Autodesk Inventor part; units mm, degrees
ref_plane "YZ Plane" through (0, 0, 0) normal (1, 0, 0) x (0, 1, 0)
ref_plane "XZ Plane" through (0, 0, 0) normal (0, 1, 0) x (-1, 0, 0)
ref_plane "XY Plane" through (0, 0, 0) normal (0, 0, 1) x (1, 0, 0)
sketch "Sketch1" plane through (0, 0, 0) normal (0, 1, 0) x (-1, 0, 0)
  circle A0 centre (0, 0) radius 1.65
  circle A1 centre (0, 0) radius 3
  circle A2 centre (5.12, 83.75) radius 1.65
  circle A3 centre (5.12, 83.75) radius 3
  circle A4 centre (93.53, 3.15) radius 1.65
  circle A5 centre (93.53, 3.15) radius 3
  line L0 (-6.58, 0) -> (-6.58, -6.22)
  line L1 (-6.58, -6.22) -> (-6.58, 91.53)
  line L2 (-6.58, 91.53) -> (103.15, 91.53)
  line L3 (103.15, 86.53) -> (103.15, -1.22)
  line L4 (103.15, -6.22) -> (-6.58, -6.22)
  line L5 (-6.58, 91.53) -> (-6.58, 88.53)
  line L6 (103.15, 91.53) -> (100.15, 91.53)
  line L7 (3, 0) -> (3, -3.22)
  line L8 (-3, 0) -> (-3, -3.22)
  line L9 (2.12, 83.75) -> (2.12, 88.53)
  line L10 (8.12, 83.75) -> (8.12, 88.53)
  line L11 (93.53, 6.15) -> (100.15, 6.15)
  line L12 (93.53, 0.15) -> (100.15, 0.15)
  line L13 (-3.58, 88.53) -> (-3.58, -3.22)
  line L14 (103.15, 91.53) -> (108.15, 91.53)
  line L15 (108.15, 91.53) -> (108.15, 86.53)
  line L16 (108.15, 86.53) -> (103.15, 86.53)
  line L17 (103.15, -6.22) -> (108.15, -6.22)
  line L18 (108.15, -6.22) -> (108.15, -1.22)
  line L19 (108.15, -1.22) -> (103.15, -1.22)
  line L20 (100.15, 88.53) -> (100.15, 6.15)
  line L21 (100.15, 0.15) -> (100.15, -3.22)
  line L22 (100.15, -3.22) -> (3, -3.22)
  line L23 (-3, -3.22) -> (-3.58, -3.22)
  line L24 (-3.58, 88.53) -> (2.12, 88.53)
  line L25 (8.12, 88.53) -> (100.15, 88.53)
  dimension "d0" = 3.3
  dimension "d1" = 6
  dimension "d4" = 3.3
  dimension "d5" = 6
  dimension "d8" = 3.3
  dimension "d9" = 6
extrude "Extrusion1" add sketch "Sketch1" against normal blind 3 contours A1 | A5 | A3 | L1 L2 L14 L15 L16 L3 L19 L18 L17 L4 L0
extrude "Extrusion2" add sketch "Sketch1" along normal blind 3 contours A1 | A5 | A3
sketch "Sketch2" plane through (0, 0, 0) normal (0, 1, 0) x (1, 0, 0)
  line L0 (-103.15, 1.22) -> (-108.15, 1.22)
  line L1 (-103.15, 1.22) -> (-103.15, 6.22)
  line L2 (-108.15, 6.22) -> (6.58, 6.22)
  line L3 (-103.15, 6.22) -> (-108.15, 6.22)
  line L4 (-108.15, 6.22) -> (-108.15, 1.22)
  line L5 (-103.15, 1.22) -> (-103.15, -86.53)
  line L6 (-108.15, 1.22) -> (-103.15, 1.22)
  line L7 (-108.15, -91.53) -> (-108.15, -86.53)
  line L8 (-108.15, -91.53) -> (-103.15, -91.53)
  line L9 (6.58, -91.53) -> (-108.15, -91.53)
  line L10 (-103.15, -86.53) -> (-103.15, -91.53)
  line L11 (-108.15, -86.53) -> (-103.15, -86.53)
  line L12 (-103.15, -86.53) -> (-108.15, -86.53)
  line L13 (-108.15, -86.53) -> (-108.15, -91.53)
  line L14 (-103.15, -91.53) -> (-104.15, -91.53)
  line L15 (-104.15, -91.53) -> (-104.15, -86.53)
  line L16 (-103.15, 1.22) -> (-104.15, 1.22)
  line L17 (-104.15, 1.22) -> (-104.15, 6.22)
  point P0 (0, 0)
  dimension "d26" = 1
  dimension "d27" = 1
extrude "Extrusion3" add sketch "Sketch2" along normal blind 41 contours L0 L4 L2 L17 | L15 L8 L7 L11
sketch "Sketch3" plane through (-104.15, 0, 91.53) normal (1, 0, 0) x (0, 0, -1)
  line L0 (0, 41) -> (5, 41)
  line L1 (0, 41) -> (0, 38)
  line L2 (0, -3) -> (0, 41)
  line L3 (0, 38) -> (5, 38)
  line L4 (5, -3) -> (5, 41)
  line L5 (5, 38) -> (5, 41)
  line L6 (5, 41) -> (0, 41)
  line L7 (92.75, 41) -> (97.75, 41)
  line L8 (92.75, 41) -> (92.75, 38)
  line L9 (92.75, -3) -> (92.75, 41)
  line L10 (92.75, 38) -> (97.75, 38)
  line L11 (97.75, -3) -> (97.75, 41)
  line L12 (97.75, 41) -> (92.75, 41)
  line L13 (97.75, 41) -> (97.75, 38)
  point P0 (91.53, 0)
  dimension "d30" = 3
  dimension "d31" = 3
extrude "Extrusion4" add sketch "Sketch3" along normal blind 35
sketch "Sketch4" plane through (0, 41, 0) normal (0, 1, 0) x (1, 0, 0)
  line L0 (-69.15, -91.53) -> (-69.15, -86.53)
  line L1 (-108.15, 1.22) -> (-69.15, 1.22)
  line L2 (-69.15, -86.53) -> (-69.15, -78.155)
  line L3 (-69.15, 1.22) -> (-69.15, -7.155)
  circle A0 centre (-74.23, -78.155) radius 1.65
  circle A1 centre (-74.23, -7.155) radius 1.65
  circle A2 centre (-92.01, -78.155) radius 1.65
  circle A3 centre (-92.01, -7.155) radius 1.65
  line L4 (-69.15, -78.155) -> (-69.15, -75.155)
  line L5 (-69.15, -75.155) -> (-69.15, -74.155)
  line L6 (-69.15, -74.155) -> (-97.09, -74.155)
  line L7 (-100.15, -88.53) -> (-100.15, -6.15)
  line L8 (-97.09, -74.155) -> (-97.09, -86.53)
  line L9 (-97.09, -86.53) -> (-69.15, -86.53)
  line L10 (-69.15, -7.155) -> (-69.15, -11.155)
  line L11 (-69.15, -11.155) -> (-97.09, -11.155)
  line L12 (-97.09, -11.155) -> (-97.09, 1.22)
  line L13 (-97.09, 1.22) -> (-69.15, 1.22)
  point P0 (0, 0)
  dimension "d46" = 3.3
  dimension "d47" = 3.3
  dimension "d50" = 3.3
  dimension "d51" = 3.3
  dimension "d53" = 1
extrude "Extrusion5" add sketch "Sketch4" against normal blind 3
sketch "Sketch5" plane through (-69.15, 0, 91.53) normal (1, 0, 0) x (0, 0, -1)
  line L0 (0, 41) -> (0, 38)
  line L1 (0, 41) -> (0, 38)
  line L2 (0, 41) -> (17.375, 41)
  line L3 (0, 41) -> (5, 41)
  line L4 (5, 41) -> (5, 38)
  line L5 (5, -3) -> (5, 41)
  line L6 (5, 38) -> (0, 38)
  line L7 (0, 38) -> (5, 38)
  line L8 (97.75, 38) -> (97.75, 41)
  line L9 (97.75, 41) -> (92.75, 41)
  line L10 (97.75, 41) -> (80.375, 41)
  line L11 (92.75, 38) -> (92.75, 41)
  line L12 (92.75, 41) -> (92.75, 38)
  line L13 (97.75, 38) -> (80.375, 38)
  line L14 (92.75, 38) -> (97.75, 38)
  line L15 (97.75, 38) -> (97.75, 41)
  point P0 (91.53, 0)
  dimension "d59" = 5
  dimension "d60" = 5
extrude "Extrusion6" add sketch "Sketch5" along normal blind 30
sketch "Sketch7" plane through (0, 41, 0) normal (0, 1, 0) x (1, 0, 0)
  line L0 (-69.15, 1.22) -> (-69.15, -11.155)
  line L1 (-69.15, 1.22) -> (-46.15, 1.22)
  line L2 (-3, 3.22) -> (-100.15, 3.22)
  line L3 (-69.15, 1.22) -> (-69.15, -11.155)
  line L4 (-69.15, -11.155) -> (-69.15, -25.405)
  line L5 (-69.15, -25.405) -> (-39.15, -25.405)
  line L6 (-39.15, 1.22) -> (-39.15, 6.22)
  line L7 (-39.15, -25.405) -> (-39.15, 1.22)
  line L8 (-39.15, 1.22) -> (-46.15, 1.22)
  circle A0 centre (-54.15, -17.905) radius 3.75
  point P0 (0, 0)
  dimension "d117" = 7.5
extrude "Extrusion8" add sketch "Sketch7" against normal blind 2
sketch "Sketch8" plane through (0, 41, 0) normal (0, 1, 0) x (1, 0, 0)
  circle A0 centre (-74.23, -78.155) radius 1.65
  circle A1 centre (-64.15, -68.155) radius 1
  circle A2 centre (-44.15, -68.155) radius 1
  circle A3 centre (-54.15, -38.155) radius 1
  line L0 (-39.15, -91.53) -> (-39.15, -86.53)
  line L1 (-39.15, -86.53) -> (-42.15, -86.53)
  line L2 (-42.15, -86.53) -> (-42.15, -39.155)
  line L3 (-42.15, -39.155) -> (-42.15, -36.155)
  line L4 (-66.15, -86.53) -> (-66.15, -36.155)
  line L5 (-66.15, -86.53) -> (-42.15, -86.53)
  line L6 (-66.15, -86.53) -> (-62.15, -86.53)
  line L7 (-69.15, -86.53) -> (-39.15, -86.53)
  line L8 (-42.15, -86.53) -> (-46.15, -86.53)
  line L9 (-62.15, -36.155) -> (-42.15, -36.155)
  line L10 (-62.15, -36.155) -> (-66.15, -36.155)
  line L11 (-46.15, -40.155) -> (-62.15, -40.155)
  line L12 (-62.15, -86.53) -> (-62.15, -40.155)
  line L13 (-46.15, -86.53) -> (-46.15, -40.155)
  point P0 (0, 0)
  dimension "d81" = 2
  dimension "d85" = 3
  dimension "d86" = 3
  dimension "d88" = 4
  dimension "d89" = 4
extrude "Extrusion9" add sketch "Sketch8" against normal blind 3 contours L5 L13 L11 L12 L4 L10 L9 L3 L2
sketch "Sketch9" plane through (0, 41, 0) normal (0, 1, 0) x (1, 0, 0)
  line L0 (-39.15, -91.53) -> (-36.15, -91.53)
  line L1 (-104.15, -91.53) -> (6.58, -91.53)
  line L2 (-36.15, -91.53) -> (-36.15, 6.22)
  line L3 (-108.15, 6.22) -> (6.58, 6.22)
  line L4 (-36.15, 6.22) -> (-39.15, 6.22)
  line L5 (-104.15, -91.53) -> (-39.15, -91.53)
  line L6 (-39.15, 6.22) -> (-39.15, -91.53)
  point P0 (0, 0)
  dimension "d94" = 3
extrude "Extrusion10" add sketch "Sketch9" against normal blind 3
sketch "Sketch10" plane through (0, 41, 0) normal (0, 1, 0) x (1, 0, 0)
  line L0 (-108.15, -86.53) -> (-103.15, -86.53)
  line L1 (-108.15, 6.22) -> (-108.15, 1.22)
  line L2 (-108.15, -86.53) -> (-108.15, 1.22)
  line L3 (-108.15, 1.22) -> (-105.15, 1.22)
  line L4 (-108.15, 1.22) -> (-97.09, 1.22)
  line L5 (-105.15, 1.22) -> (-105.15, -86.53)
  line L6 (-103.15, 1.22) -> (-103.15, -86.53)
  line L7 (-105.15, -86.53) -> (-108.15, -86.53)
  point P0 (0, 0)
  dimension "d97" = 3
extrude "Extrusion11" add sketch "Sketch10" against normal blind 3 contours L2 L3 L5 L0
sketch "Sketch11" plane through (0, 41, 0) normal (0, 1, 0) x (1, 0, 0)
  line L0 (-86.93, -78.155) -> (-86.93, -86.53)
  line L1 (-79.31, -78.155) -> (-79.31, -86.53)
  line L2 (-79.31, -86.53) -> (-86.93, -86.53)
  line L3 (-79.31, -78.155) -> (-79.31, -74.155)
  line L4 (-79.31, -74.155) -> (-86.93, -74.155)
  line L5 (-86.93, -78.155) -> (-86.93, -74.155)
  line L6 (-86.93, -7.155) -> (-86.93, 0)
  line L7 (-79.31, -7.155) -> (-79.31, 0)
  line L8 (-79.31, 0) -> (-86.93, 0)
  line L9 (-79.31, -7.155) -> (-79.31, -11.155)
  line L10 (-86.93, -7.155) -> (-86.93, -11.155)
  line L11 (-86.93, -11.155) -> (-79.31, -11.155)
  line L12 (-47.07, -17.905) -> (-47.07, 0)
  line L13 (-61.95, -17.905) -> (-61.95, 0)
  line L14 (-61.95, -17.905) -> (-61.95, -25.405)
  line L15 (-69.15, -25.405) -> (-39.15, -25.405)
  line L16 (-61.95, -25.405) -> (-47.07, -25.405)
  line L17 (-47.07, -25.405) -> (-47.07, -17.905)
  line L18 (-61.95, -25.405) -> (-69.15, -25.405)
  line L19 (-69.15, -25.405) -> (-69.15, 0)
  line L20 (-69.15, 1.22) -> (-69.15, -11.155)
  line L21 (-61.95, 0) -> (-69.15, 0)
  line L22 (-47.07, -25.405) -> (-39.15, -25.405)
  line L23 (-39.15, -25.405) -> (-39.15, 0)
  line L24 (-39.15, 0) -> (-47.07, 0)
  line L25 (-54.15, -17.905) -> (-54.15, -25.405)
  line L26 (-39.15, -25.405) -> (-69.15, -25.405)
  line L27 (-54.15, -25.405) -> (-54.15, -17.905)
  line L28 (-54.15, -17.905) -> (-54.15, -10.405)
  line L29 (-54.15, -10.405) -> (-58.15, -10.405)
  line L30 (-58.15, -10.405) -> (-58.15, 0)
  line L31 (-58.15, 0) -> (-50.15, 0)
  line L32 (-50.15, 0) -> (-50.15, -10.405)
  line L33 (-50.15, -10.405) -> (-54.15, -10.405)
  point P0 (0, 0)
  point P1 (-92.01, -78.155)
  point P2 (-74.23, -78.155)
  point P3 (-92.01, -7.155)
  dimension "d111" = 7.5
  dimension "d112" = 7.5
  dimension "d113" = 4
  dimension "d114" = 8
extrude "Extrusion12" cut sketch "Sketch11" against normal blind 10
properties part number "electronic_holder"
Can you work these out from the model? Positions are in its coordinate system, mm. A direction names the side the tool comes from. Give positions to 0.01 mm unless a question says otherwise; leave off trailing zeros. Order: outer loops, then holes, each group sorted by start corner. A loop starts at its lowest first (then second) coordinate and runs counter-clockwise, first axis right, second up. Notation, with made-up numbers: M 15,71 L 39,71 A25 cw 39,105 Z; hole C -14,-34 d5. An arc over 180 degrees is marked long. Use one line per item in the form item = value.
Item 1: If I drill on line 1 along Z through (x, y) = (-93.53, -0.4); line 2 along X through (y, z) = (39, 55.5); line 3 along Z through (x, y) = (-92, 39) (3 decimals), over which ranges is the centre line in solid material (lowest first)? Write a range as [from, to].
Values follow:
line_1 = [-6.22, -3.22], [0.15, 1.5], [4.8, 6.15], [88.53, 91.53]
line_2 = [-108.15, -105.15], [-66.15, -62.15], [-46.15, -42.15], [-39.15, -36.15]
line_3 = [-6.22, 5.505], [8.805, 11.155], [74.155, 76.505], [79.805, 91.53]
Item 2: If we section it at A-A, the plane y = 36.5: Write out the boundary of the cut face in (x, z).
Values follow:
outline = M -108.15,-6.22 L -104.15,-6.22 L -104.15,-1.22 L -108.15,-1.22 Z; M -108.15,86.53 L -104.15,86.53 L -104.15,91.53 L -108.15,91.53 Z
Item 3: Thinking about a two-plate mould opening in X: for faces 1 (the flat face through (-1.3, 3, -1.3)), 2 (the flat face through (-105.15, 40, 42)), which applies, pulls with the +X half, pulls with the -X half, needs draft (parallel to the pull), parting line crosses it, or undercut?
Values follow:
face_1 = needs draft
face_2 = undercut
Item 4: Will these pins go through, and if not, where does the flat tip stop? pin 1 Ø2.5 at (y, z) = (39.5, 79.5) entering from +X; pin 2 Ø4.5 at (x, z) = (-74.23, 7.155) entering from +Y; pin 3 Ø12 at (x, z) = (-54.15, 17.905) entering from -Y; pin 4 Ø0.9 at (x, z) = (-106.5, 38.5) entering from -Y.
Values follow:
pin_1 = -36.15
pin_2 = 41
pin_3 = 39
pin_4 = 38
Item 5: If we section it at D-D, the plane x = -5.12: Write out the boundary of the cut face in (y, z).
Values follow:
outline = M -3,-6.22 L 0,-6.22 L 0,-3.22 L -3,-3.22 Z; M -3,80.75 L 3,80.75 L 3,82.1 L -3,82.1 Z; M -3,85.4 L 3,85.4 L 3,86.75 L 0,86.75 L 0,91.53 L -3,91.53 Z
Item 6: If we section it at C-C, the plane z = 59: Write out the boundary of the cut face in (x, y), and give its area (3 significant figures).
Values follow:
outline = M -108.15,38 L -105.15,38 L -105.15,41 L -108.15,41 Z; M -103.15,-3 L -100.15,-3 L -100.15,0 L -103.15,0 Z; M -66.15,38 L -62.15,38 L -62.15,41 L -66.15,41 Z; M -46.15,38 L -42.15,38 L -42.15,41 L -46.15,41 Z; M -39.15,38 L -36.15,38 L -36.15,41 L -39.15,41 Z; M 3.58,-3 L 6.58,-3 L 6.58,0 L 3.58,0 Z
area = 60.0 mm^2
Item 7: If we section it at B-B, the plane x = -74.23: Write out the boundary of the cut face in (y, z) (3 decimals).
Values follow:
outline = M -3,-6.22 L 0,-6.22 L 0,-3.22 L -3,-3.22 Z; M -3,88.53 L 0,88.53 L 0,91.53 L -3,91.53 Z; M 38,-6.22 L 41,-6.22 L 41,5.505 L 38,5.505 Z; M 38,8.805 L 41,8.805 L 41,11.155 L 38,11.155 Z; M 38,74.155 L 41,74.155 L 41,76.505 L 38,76.505 Z; M 38,79.805 L 41,79.805 L 41,91.53 L 38,91.53 Z
Item 8: For faces 3 (the flat face through (-52, -1, -3.22)), 4 (the flat face through (-107, 38, 42)), 5 (the flat face through (-68, -0.5, -6.22)), 6 (the flat face through (-42.15, 40, 62)), 7 (the cylindrical face through (-93.226, 39.521, 6.04)), which set-ups out of +Z, -Z, +X, -X, +Y, -Y let a thin tool reach every point of the face, with its end or its side?
Values follow:
face_3 = -Y
face_4 = +X, -X, -Y
face_5 = -Z, +X, -X, +Y, -Y
face_6 = +Y, -Y
face_7 = +Y
